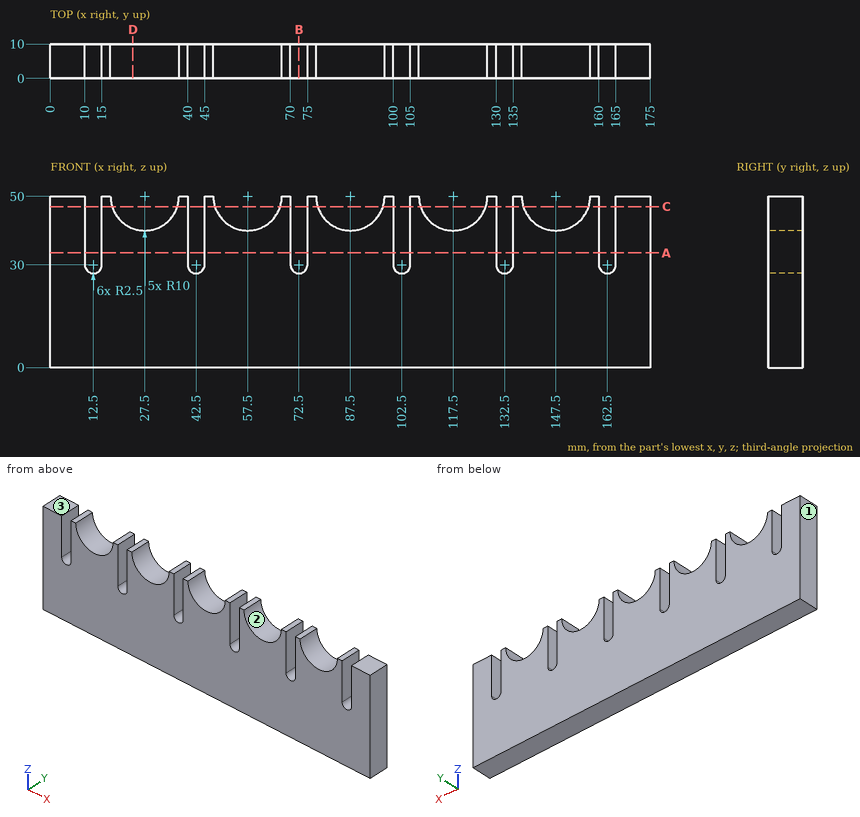
Could you check a few things on this drawing? It's one solid part, dimensions in mm from its lowest x, y, z. Coordinates: 2 decimals unless noted, no trailing zeros. Order: outer loops, then holes, each group sorted by start corner. A loop starts at its lowest first (then second) coordinate and runs counter-clockwise, first axis right, second up. Notation, with made-up numbers: M -9.75,40 L 37.25,40 A21 ccw 37.25,53 Z; hole C 53,-35.75 d3. An arc over 180 degrees is marked long. Answer as a JSON object with one key per item and string values. Group by question number.
(1) Suppose I cut it at A-A, the plane z = 33.5. Please give me the cut outline in (x, y), then the cut area to 3 significant figures.
(2) Suppose I cut it at D-D, the plane x = 24. Please give me the cut outline in (y, z).
(3) For pin 1 (3 mm diameter, centred on x = 56.5, y = 2.5, fed in from -Z), with a flat end and sliding along its axis, tell me the tip position at first contact or that it passes through.
(4) I need wall thicknesses on probe 1 along Z at (x, y) = (12.5, 3); probe 2 along Z at (x, y) = (147.5, 9.5). Which ranges of each line are inside material? Lowest first, please.
(5) Suppose I cut it at C-C, the plane z = 47. State how many separate pieces and enclosed holes the cut face has, then the cut area to 3 significant figures.
(6) Suppose I cut it at B-B, the plane x = 72.5. Please give me the cut outline in (y, z).
(7) If we mould it in two halves opening along X, with no side actions, what happens to the marked faces 1, 2 and 3? For each: released by +X, released by -X, zero draft, split by the parting line, or undercut.
Values found:
{
 "1": {"outline": "M 0,0 L 10,0 L 10,10 L 0,10 Z; M 15,0 L 40,0 L 40,10 L 15,10 Z; M 45,0 L 70,0 L 70,10 L 45,10 Z; M 75,0 L 100,0 L 100,10 L 75,10 Z; M 105,0 L 130,0 L 130,10 L 105,10 Z; M 135,0 L 160,0 L 160,10 L 135,10 Z; M 165,0 L 175,0 L 175,10 L 165,10 Z", "area": "1,450 mm^2"},
 "2": {"outline": "M 0,0 L 10,0 L 10,40.63 L 0,40.63 Z"},
 "3": {"pin 1": "stops at z = 0"},
 "4": {"probe 1": "z = 0 to 27.5", "probe 2": "z = 0 to 40"},
 "5": {"separate pieces": "12", "enclosed holes": "0", "area": "496 mm^2"},
 "6": {"outline": "M 0,0 L 10,0 L 10,27.5 L 0,27.5 Z"},
 "7": {"face 1": "released by -X", "face 2": "undercut", "face 3": "zero draft"}
}
